Work out the finished part from the listing and answer in its coordinate system (mm). A direction names the side the tool comes from. Give positions to 0.01 mm unless a question says otherwise; leave off trailing zeros. Order: outer loops, then holes, each group sorted by start corner. A loop starts at its lowest first (then second) coordinate and runs counter-clockwise, first axis right, second up. Notation, with made-up numbers: (5, 10) -> (10, 10) arc R27 ccw to (10, 41) -> close; hole circle Ø1 at (73.5, 4). An arc over 180 degrees is marked (long way). Use a Markdown table: item, result. Add a question column.
Autodesk Inventor part; units mm, degrees
ref_plane "YZ Plane" through (0, 0, 0) normal (1, 0, 0) x (0, 1, 0)
ref_plane "XZ Plane" through (0, 0, 0) normal (0, 1, 0) x (-1, 0, 0)
ref_plane "XY Plane" through (0, 0, 0) normal (0, 0, 1) x (1, 0, 0)
sketch "Skizze1" plane through (0, 0, 0) normal (0, 0, 1) x (1, 0, 0)
  line L0 (-82.5, 125) -> (82.5, 125)
  line L1 (82.5, 125) -> (82.5, -125)
  line L2 (82.5, -125) -> (-82.5, -125)
  line L3 (-82.5, -125) -> (-82.5, 125)
  line L4 (-82.5, 125) -> (82.5, -125) construction
  line L5 (82.5, 125) -> (-82.5, -125) construction
  point P0 (0, 0)
  dimension "d0" = 165
  dimension "d1" = 250
extrude "Extrusion1" add sketch "Skizze1" along normal blind 70
sketch "Skizze2" plane through (0, 0, 0) normal (0, 0, -1) x (-1, 0, 0)
  line L0 (82.5, 125) -> (-82.5, 125)
  circle A0 centre (0, 37.5) radius 52.5
  point P0 (0, 0)
  dimension "d4" = 105
  dimension "d5" = 35
extrude "Extrusion2" add sketch "Skizze2" along normal blind 10
chamfer "Fase1" distance 30 angle 60 1 edges at (0, -125, 0) measured on face at (27.5, -125, 23.3333)
sketch "Skizze3" plane through (0, 0, 70) normal (0, 0, 1) x (1, 0, 0)
  line L0 (82.5, 125) -> (-82.5, 125)
  line L1 (-82.5, 125) -> (-82.5, -125)
  line L2 (-82.5, -125) -> (82.5, -125)
  line L3 (82.5, -125) -> (82.5, 125)
  line L4 (-82.5, -115) -> (82.5, -115)
  point P0 (0, 0)
  dimension "d11" = 10
ref_plane "Arbeitsebene1" through (-82.5, -115, 70) normal (0, 0.1736, 0.9848) x (1, 0, 0)
sketch "Skizze4" plane through (0, 0, 70) normal (0, 0, 1) x (1, 0, 0)
  line L0 (82.5, 125) -> (-82.5, 125)
  line L1 (-82.5, 125) -> (-82.5, -125)
  line L2 (82.5, -125) -> (82.5, 125)
  line L3 (-70, -115) -> (70, -115) construction
  line L4 (70, -115) -> (70, 115)
  line L5 (70, 115) -> (-70, 115)
  line L6 (-70, 115) -> (-70, -115)
  line L7 (-70, -115) -> (70, 115) construction
  line L8 (70, -115) -> (-70, 115) construction
  line L9 (-82.5, -115) -> (82.5, -115)
  point P0 (0, 0)
  point P1 (0, 0)
  point P2 (0, 0)
  dimension "d13" = 230
  dimension "d14" = 140
extrude "Extrusion3" cut sketch "Skizze4" against normal up to surface contours L2 L9 L4 L5 L6 L1 L0 surface through (-82.5, -115, 70) normal (0, 0.1736, 0.9848)
sketch "Skizze5" plane through (0, 0, 70) normal (0, 0, 1) x (1, 0, 0)
  line L0 (82.5, -115) -> (70, -115)
  line L1 (70, -115) -> (70, 115)
  line L2 (70, 115) -> (-70, 115)
  line L3 (-70, 115) -> (-70, -115)
  line L4 (-70, -115) -> (-82.5, -115)
  line L5 (-82.5, -115) -> (-82.5, -125)
  line L6 (-82.5, -125) -> (82.5, -125)
  line L7 (82.5, -125) -> (82.5, -115)
  line L8 (55, 100) -> (-55, 100) construction
  line L9 (-55, 100) -> (-55, -100) construction
  line L10 (-55, -100) -> (55, -100) construction
  line L11 (55, -100) -> (55, 100) construction
  line L12 (55, 100) -> (-55, -100) construction
  line L13 (-55, 100) -> (55, -100) construction
  circle A0 centre (-55, -100) radius 15
  circle A1 centre (-55, 100) radius 15
  circle A2 centre (55, 100) radius 15
  circle A3 centre (55, -100) radius 15
  line L14 (-82.5, -115) -> (-82.5, 125)
  line L15 (-70, -115) -> (-82.5, -115)
  line L16 (-70, 115) -> (-70, -115)
  line L17 (70, 115) -> (-70, 115)
  line L18 (70, -115) -> (70, 115)
  line L19 (82.5, -115) -> (70, -115)
  line L20 (82.5, 125) -> (82.5, -115)
  line L21 (-82.5, 125) -> (82.5, 125)
  point P0 (0, 0)
  dimension "d17" = 110
  dimension "d18" = 200
  dimension "d19" = 30
extrude "Extrusion4" cut sketch "Skizze5" against normal blind 5 contours L7 L6 L5 L4 L3 A1 L2 A2 L1 L0 | L0 L1 L2 L3 L4 L14 L21 L20 | A2 L2 L1 | A1 L3 L2
properties part number "Scale" material "Blei"
1) Flat-ended cylindrical pins translate along their axes: pin 1 (1.5 mm diameter, centred on y = 35.5, z = 54.5, fed in from +X); pin 2 (1.5 mm diameter, centred on x = -0.5, z = 46.5, fed in from +Y); pin 3 (5 mm diameter, centred on x = 32, y = -64.5, fed in from +Z); pin 4 (6 mm diameter, centred on x = 58.5, z = 28, fed in from -Y). Find the tip coordinate at first contact, or state that the pin passes through.
2) The part is cut by section D-D, the plane x = 0. Determine the outline of the cut face in (y, z).
3) Which of the six approach directions +Z, -Z, +X, -X, +Y, -Y give full straight-line access (tool end or side, diameter ignored) to faces 1 (the flat face through (1, 115, 47)), 2 (the flat face through (-70, 38, 51)), 3 (the flat face through (70, 58, 55)), 4 (the cylindrical face through (11.38, 88.75, -4.93)), 5 (the flat face through (-1, -3, 65))?
4) The part is cut by section B-B, the plane y = -96. Determine the outline of the cut face in (x, z), then the cut area to 3 significant figures.
5) The part is cut by section A-A, the plane x = -64. Determine the outline of the cut face in (y, z).
6) Determine the mould class of faces 6 (the flat face through (-1.155, -98.656, 14.79)), 7 (the flat face through (-1, 125, 14)), 8 (the flat face through (-55, -100, 70)) for opening direction Z: released by +Z, released by -Z, zero draft, split by the parting line, or undercut.
7) The part is cut by section C-C, the plane z = 40. Determine the outline of the cut face in (x, y), then the cut area to 3 significant figures.
8) Straight lines are drawn through the part: line 1 (Y direction, x = -5.5, z = 58); line 2 (X direction, y = -44.5, z = 59.5); line 3 (Z direction, x = -30, y = -1.5). For each, find the intervals that lie inside material, in ascending order.
A:
| question | item | result |
|---|---|---|
| 1 | pin 1 | x = 70 |
| 1 | pin 2 | y = 115 |
| 1 | pin 3 | z = 65 |
| 1 | pin 4 | y = -125 |
| 2 | outline | (-125, 30) -> (-73.04, 0) -> (-15, 0) -> (-15, -10) -> (90, -10) -> (90, 0) -> (125, 0) -> (125, 27.68) -> (115, 29.44) -> (115, 65) -> (-125, 65) -> close |
| 3 | face 1 | +Z, +X, -X, +Y |
| 3 | face 2 | +Z, -X, +Y |
| 3 | face 3 | +Z, +X, +Y |
| 3 | face 4 | -Z |
| 3 | face 5 | +Z |
| 4 | outline | (-82.5, 13.26) -> (82.5, 13.26) -> (82.5, 65) -> (69.46, 65) -> (69.46, 70) -> (40.54, 70) -> (40.54, 65) -> (-40.54, 65) -> (-40.54, 70) -> (-69.46, 70) -> (-69.46, 65) -> (-82.5, 65) -> close |
| 4 | area | 8,830 mm^2 |
| 5 | outline | (-125, 30) -> (-73.04, 0) -> (125, 0) -> (125, 27.68) -> (115, 29.44) -> (115, 65) -> (112, 65) -> (112, 70) -> (88, 70) -> (88, 65) -> (-88, 65) -> (-88, 70) -> (-112, 70) -> (-112, 65) -> (-125, 65) -> close |
| 6 | face 6 | released by -Z |
| 6 | face 7 | zero draft |
| 6 | face 8 | released by +Z |
| 7 | outline | (-82.5, -125) -> (82.5, -125) -> (82.5, 55.14) -> (70, 55.14) -> (70, 115) -> (-70, 115) -> (-70, 55.14) -> (-82.5, 55.14) -> close |
| 7 | area | 38,100 mm^2 |
| 8 | line 1 | -125 to 115 |
| 8 | line 2 | -70 to 70 |
| 8 | line 3 | -10 to 65 |
